from build123d import *

# Parameters (mm, degrees)
F0_W     = 60
F0_H     = 60
F1_DEPTH = 60
F2_W     = 15
F2_H     = 15
F3_DEPTH = 30
F4_R     = 12.5
F5_DEPTH = 60


with BuildPart() as f1:
    # F0 (on Top) → F1 (new body)
    with BuildSketch(Plane.XY):
        Rectangle(F0_W, F0_H)
    extrude(amount=F1_DEPTH)

    # F2 (on face) → F3 (join)
    with BuildSketch(Plane.XY.offset(60)):
        with Locations((-22.5, -22.5)):
            Rectangle(F2_W, F2_H)
        with Locations((-22.5, 22.5)):
            Rectangle(F2_W, F2_H)
        with Locations((22.5, 22.5)):
            Rectangle(F2_W, F2_H)
        with Locations((22.5, -22.5)):
            Rectangle(F2_W, F2_H)
    extrude(amount=F3_DEPTH)

    # F4 (on face) → F5 (cut)
    with BuildSketch(Plane.XY.offset(60)):
        Circle(F4_R)
    extrude(amount=-F5_DEPTH, mode=Mode.SUBTRACT)


solid = f1.part
CAD build for the part. Positions are in the model's coordinates, mm. A direction names the side the tool comes from. Round coordinates to 2 decimals unless told otherwise and drop trailing zeros. Write each loop counter-clockwise with the first axis right and the second up, starting at its lowest first coordinate (ties: lowest second). Pieces come first, ordered by that corner, then holes.
(1) Slice it at D-D, the plane z = 32. Write the cut outline in (x, y).
(2) 3-axis set-ups, long thin cutter, end or side, ignore diameter. For faces 4 (the face through (11.923, 3.755, 30.42)), 5 (the face through (15, 22, 75)), 6 (the face through (22, -15, 75)): which of +Z, -Z, +X, -X, +Y, -Y reach the whole face in a straight line?
(3) Slice it at A-A, the plane y = 0. Write the cut outline in (x, z), and give its area (3 significant figures).
(4) Mould opens along X. For faces 1 (the face through (-30, 0, 34)), 2 (the face through (-15, -23, 75)), 3 (the face through (22, 15, 75)) say: pulls with the +X half, pulls with the -X half, needs draft (parallel to the pull), parting line crosses it, or undercut.
(5) Probe line 1 along Y through (x, z) = (0, 13); line 2 along Y through (x, z) = (-26, 85.5); line 3 along Z through (x, y) = (13, -24). List the from-to ranges inside material, lowest first.
(6) Drop a flat-ended pin along its axis: P1, Ø2, axis at x = -10.5, y = -20.5, coming from the +Z side. Give the stop position or say it passes through.
(7) Slice it at B-B, the plane z = 63.5. Write the cut outline in (x, y).
(8) Slice it at C-C, the plane x = -10. Write the cut outline in (y, z), and give its area (3 significant figures).
From the geometry:
1. outline: (-30, -30) - (30, -30) - (30, 30) - (-30, 30) - close; hole circle Ø25 at (0, 0)
2. face 4: +Z, -Z
2. face 5: +Z, +Y, -Y
2. face 6: +Z, +X, -X
3. outline: (-30, 0) - (-12.5, 0) - (-12.5, 60) - (-30, 60) - close; (12.5, 0) - (30, 0) - (30, 60) - (12.5, 60) - close
3. area: 2,100 mm2
4. face 1: pulls with the -X half
4. face 2: undercut
4. face 3: needs draft
5. line 1: y = -30 to -12.5, 12.5 to 30
5. line 2: y = -30 to -15, 15 to 30
5. line 3: z = 0 to 60
6. P1: stops at z = 60
7. outline: (-30, -30) - (-15, -30) - (-15, -15) - (-30, -15) - close; (-30, 15) - (-15, 15) - (-15, 30) - (-30, 30) - close; (15, -30) - (30, -30) - (30, -15) - (15, -15) - close; (15, 15) - (30, 15) - (30, 30) - (15, 30) - close
8. outline: (-30, 0) - (-7.5, 0) - (-7.5, 60) - (-30, 60) - close; (7.5, 0) - (30, 0) - (30, 60) - (7.5, 60) - close
8. area: 2,700 mm2
